Answer from the drawing. Dimensions are ordinates in mm from the lowest x, y and z of the part. A direction names the side the tool comes from. Give positions to 0.01 mm unless a question says otherwise; leave off trailing zeros. Loops run counter-clockwise (first coordinate to the right, second up) from the corner with the lowest first, then second, coordinate; pieces in that order, holes last.
(1) Find section B-B, the plane z = 3.5. Write down the section's boundary in (x, y), then the cut area to 3 significant figures.
(2) Straight lines are drawn through the part: probe 1 along X at (y, z) = (1.85, 8); probe 2 along X at (y, z) = (11, 3); probe 3 along X at (y, z) = (1.5, 6.75). For each, find the intervals that lie inside material, in ascending order.
(3) Which of the six approach directions +Z, -Z, +X, -X, +Y, -Y give full straight-line access (tool end or side, diameter ignored) to the marked faces 1, 2 and 3?
(4) Find section C-C, the plane y = 16. Write down the section's boundary in (x, z), then the cut area to 3 significant figures.
(5) Determine the mould class of the marked faces 4, 5 and 6 for opening direction Z: pulls with the +Z half, pulls with the -Z half, needs draft (parallel to the pull), parting line crosses it, or undercut.
(6) Each of these flat-tipped pins is pushed along its axis until it touches: P1, Ø1.2, axis at x = 18.5, z = 1.5, coming from the +Y side; P2, Ø3, axis at x = 16.5, z = 7.5, coming from the +Y side; P3, Ø2, axis at x = 15, y = 7.5, coming from the +Z side. Where does it stop, or does it pass through?
(7) Find section D-D, the plane z = 8. Write down the section's boundary in (x, y).
(8) Find section A-A, the plane y = 12.5. Write down the section's boundary in (x, z).
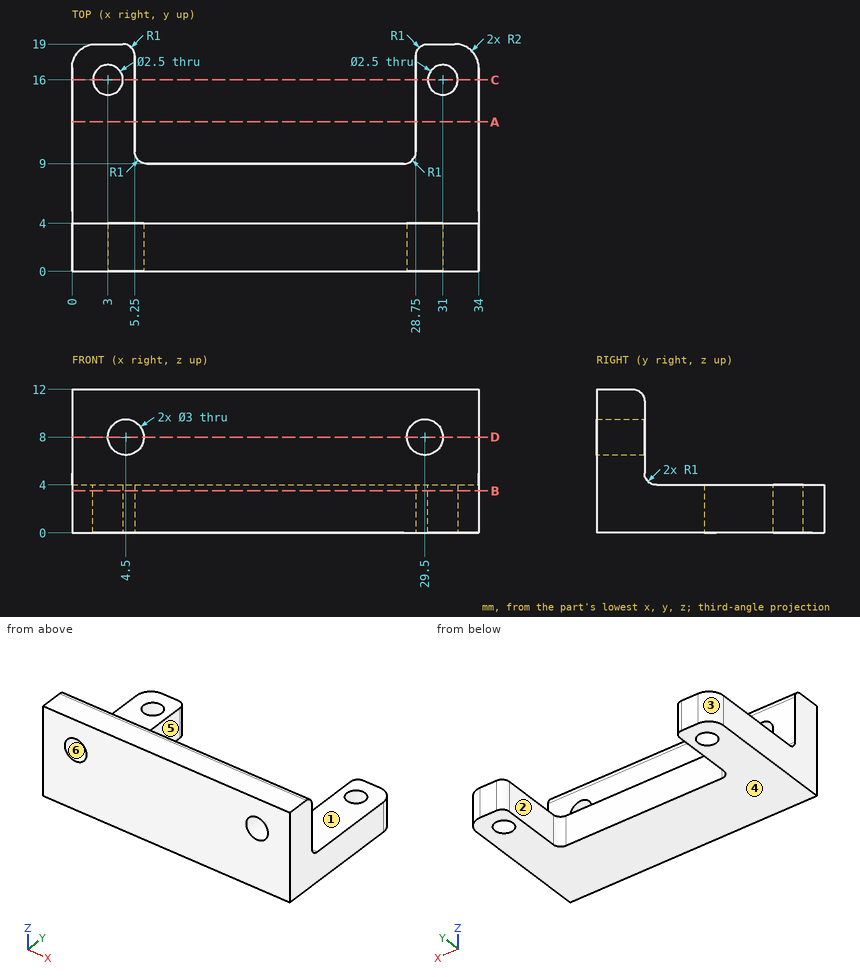
Entries:
1. outline: (0, 0) - (34, 0) - (34, 17) arc R2 ccw to (32, 19) - (29.75, 19) arc R1 ccw to (28.75, 18) - (28.75, 10) arc R1 cw to (27.75, 9) - (6.25, 9) arc R1 cw to (5.25, 10) - (5.25, 18) arc R1 ccw to (4.25, 19) - (2, 19) arc R2 ccw to (0, 17) - close; hole circle Ø2.5 at (3, 16); hole circle Ø2.5 at (31, 16)
1. area: 399 mm2
2. probe 1: x = 0 to 3, 6 to 28, 31 to 34
2. probe 2: x = 0 to 5.25, 28.75 to 34
2. probe 3: x = 0 to 3.67, 5.33 to 28.67, 30.33 to 34
3. face 1: +Z, +X, -X, +Y
3. face 2: +Z, -Z, +Y
3. face 3: +Z, -Z, -X, +Y
4. outline: (0, 0) - (1.75, 0) - (1.75, 4) - (0, 4) - close; (4.25, 0) - (5.25, 0) - (5.25, 4) - (4.25, 4) - close; (28.75, 0) - (29.75, 0) - (29.75, 4) - (28.75, 4) - close; (32.25, 0) - (34, 0) - (34, 4) - (32.25, 4) - close
4. area: 22.0 mm2
5. face 4: pulls with the -Z half
5. face 5: needs draft
5. face 6: undercut
6. P1: stops at y = 9
6. P2: stops at y = 4
6. P3: stops at z = 4
7. outline: (0, 0) - (3, 0) - (3, 4) - (0, 4) - close; (6, 0) - (28, 0) - (28, 4) - (6, 4) - close; (31, 0) - (34, 0) - (34, 4) - (31, 4) - close
8. outline: (0, 0) - (5.25, 0) - (5.25, 4) - (0, 4) - close; (28.75, 0) - (34, 0) - (34, 4) - (28.75, 4) - close
